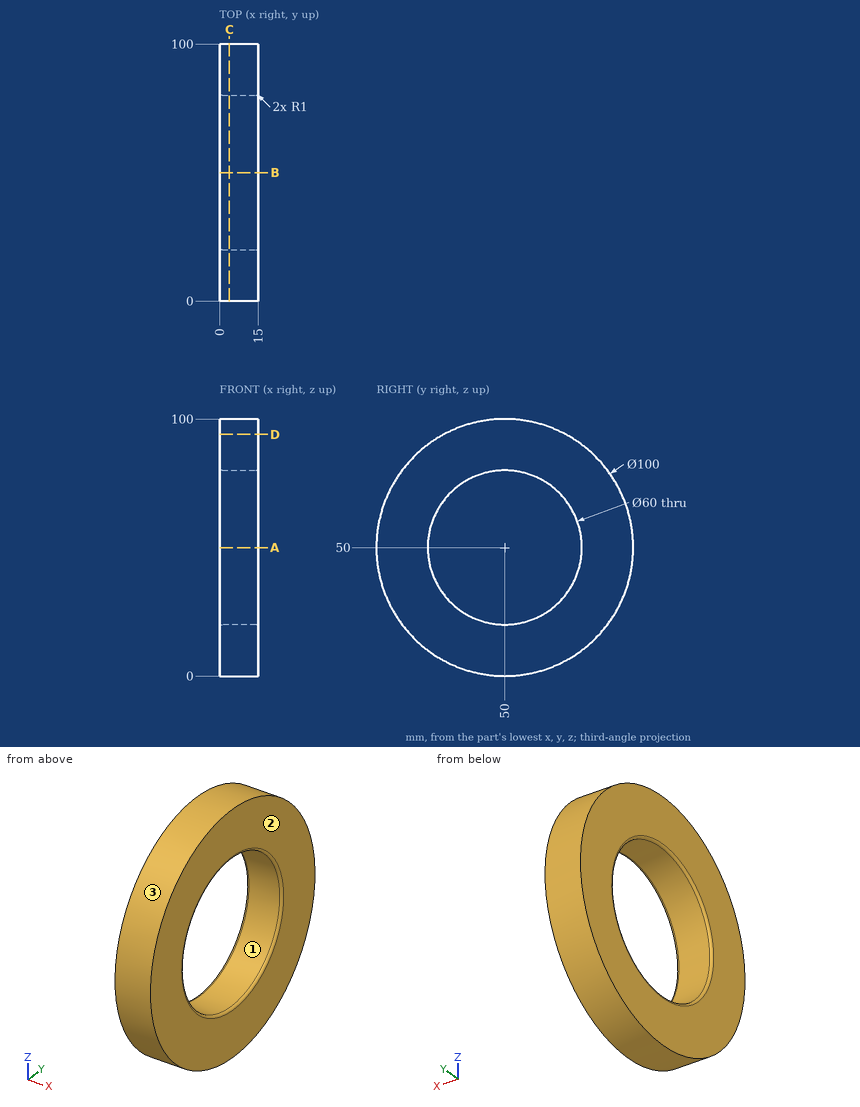
Geometry check sheet. Reference: drawing and pictorial views, mm from the part's lowest x, y, z. Round coordinates to 2 decimals unless told otherwise and drop trailing zeros. Loops run counter-clockwise (first coordinate to the right, second up) from the corner with the lowest first, then second, coordinate; pieces in that order, holes last. Notation, with made-up numbers: (54.25, 54.25) - (76.25, 54.25) arc R21 cw to (76.25, 88.25) - close; hole circle Ø1 at (13.25, -15.75). An arc over 180 degrees is marked (long way). One line per question, with ' | ' between items. Start each with the question number.
1. Draft check along Z on the marked faces 1, 2 and 3. Enter one of: released by +Z, released by -Z, zero draft, split by the parting line, or undercut.
2. Cross-section at D-D on z = 94. Record the cut outline in (x, y), then the cut area to 3 significant figures.
3. Cross-section at C-C on x = 3.75. Record the cut outline in (y, z), then the cut area to 3 significant figures.
4. Cross-section at A-A on z = 50. Record the cut outline in (x, y).
5. Scan lines: line 1 (Y direction, x = 10.5, z = 50); line 2 (Z direction, x = 8, y = 51); line 3 (Z direction, x = 8.25, y = 69). Record each from-to range of solid material in increasing order. Write a range as [from, to].
6. Depth check by flat-ended pin: pin 1 (2 mm diameter, centred on x = 1.5, z = 12, fed in from +Y); pin 2 (1.5 mm diameter, centred on y = 79, z = 48.5, fed in from -X); pin 3 (6 mm diameter, centred on x = 2, y = 86.5, fed in from +Z); pin 4 (8 mm diameter, centred on x = 5, z = 61, fed in from -Y). Enter the tip coordinate at first touch or a pass-through.
Taken from the geometry:
1) face 1: undercut | face 2: zero draft | face 3: split by the parting line
2) outline: (0, 26.25) - (15, 26.25) - (15, 73.75) - (0, 73.75) - close | area: 712 mm²
3) outline: circle Ø100 at (50, 50); hole circle Ø60 at (50, 50) | area: 5,030 mm²
4) outline: (0, 0) - (15, 0) - (15, 19) arc R1 ccw to (14, 20) - (1, 20) arc R1 ccw to (0, 19) - close; (0, 81) arc R1 ccw to (1, 80) - (14, 80) arc R1 ccw to (15, 81) - (15, 100) - (0, 100) - close
5) line 1: [0, 20], [80, 100] | line 2: [0.01, 20.02], [79.98, 99.99] | line 3: [3.75, 26.78], [73.22, 96.25]
6) pin 1: y = 83.63 | pin 2: through | pin 3: z = 87.12 | pin 4: y = 0.49
